Input: part model. Units: mm. Frame: model coordinates. A direction names the side the tool comes from. Round coordinates to 2 decimals unless told otherwise and drop trailing zeros. Loops run counter-clockwise (first coordinate to the right, second up) from the corner with the lowest first, then second, coordinate; pieces in that order, holes last.
1) Section A-A, the plane z = -59. Return loops of the section in (x, y), and give its area (3 significant figures).
2) Ray query, line 1 along Z through (x, y) = (-60.5, 0.5); line 2 along X through (y, z) = (-1, -37.5); line 3 along Z through (x, y) = (55.5, 4.75). Return the intervals inside material, ascending.
3) Section C-C, the plane y = -3.25. State how many separate pieces and enclosed holes the cut face has, and give its area (3 significant figures).
4) Draft query along Z for faces 1 (the face through (42, 4, -31)), 2 (the face through (-14, 5, -61)), 3 (the face through (-16, 6.25, -51)). Return one class per face: pulls with the +Z half, pulls with the -Z half, needs draft (parallel to the pull), parting line crosses it, or undercut.
5) First-contact query: pin 1 (4 mm diameter, centred on x = 57.5, y = 6.5, fed in from -Z); pin 2 (10 mm diameter, centred on x = -5.5, y = -2, fed in from +Z); pin 3 (2 mm diameter, centred on x = 34.5, z = -3, fed in from +Y). Flat tips, straight axial feed; report the tip coordinate or a pass-through.
6) Section D-D, the plane x = -1.5. Return loops of the section in (y, z).
7) Access query for faces 4 (the face through (-51.5, -1, 36)), 5 (the face through (48.95, 7, -30)), 6 (the face through (-11, 4, -66)). Directions: +Z, -Z, +X, -X, +Y, -Y. A direction counts if a zero-diameter tool reaches every point of the face in a straight line with its end or side. Return the directions, or none.
8) Section B-B, the plane x = 55.5. Return loops of the section in (y, z), and give its area (3 significant figures).
from build123d import *

# Parameters (mm, degrees)
SKETCH1_W           = 141
SKETCH1_H           = 82
BOSS_EXTRUDE1_DEPTH = 9
SKETCH3_R           = 2
CUT_EXTRUDE1_DEPTH  = 19
SKETCH4_W           = 8.7
SKETCH4_H           = 13.5
CUT_EXTRUDE2_DEPTH  = 10
SKETCH5_W           = 20
SKETCH5_H           = 5
CUT_EXTRUDE3_DEPTH  = 10
SKETCH6_W           = 3.23
SKETCH6_H           = 5.77
BOSS_EXTRUDE2_DEPTH = 3.3
SKETCH7_R           = 2.425
BOSS_EXTRUDE3_DEPTH = 20
LPATTERN1_COUNT     = 3
LPATTERN1_PITCH     = 31.7
SKETCH8_W           = 8.5
SKETCH8_H           = 5
SKETCH8_H_2         = 0.25
BOSS_EXTRUDE4_DEPTH = 30
SKETCH10_R          = 2.225
BOSS_EXTRUDE6_DEPTH = 5
LPATTERN2_COUNT     = 3
LPATTERN2_PITCH     = 31
SKETCH9_W           = 12
SKETCH9_H           = 5
SKETCH9_W_2         = 10
SKETCH9_W_3         = 5
SKETCH9_H_2         = 8
SKETCH9_H_3         = 18.5
SKETCH9_H_4         = 16.5
SKETCH9_W_4         = 8.75
SKETCH9_W_5         = 14
CUT_EXTRUDE4_DEPTH  = 5


with BuildPart() as part:
    # Sketch1 → Boss-Extrude1 (new body, symmetric)
    with BuildSketch(Plane(origin=(0, 0, 0), x_dir=(1, 0, 0), z_dir=(0, 1, 0))):
        Rectangle(SKETCH1_W, SKETCH1_H)
    extrude(amount=BOSS_EXTRUDE1_DEPTH, both=True)

    # Sketch3 → Cut-Extrude1 (cut, through all)
    with BuildSketch(Plane(origin=(0, 9, 0), x_dir=(1, 0, 0), z_dir=(0, 1, 0))):
        with Locations((-60.5, 37.5)):
            Circle(SKETCH3_R)
        with Locations((-1.5, 37.5)):
            Circle(SKETCH3_R)
        with Locations((55.5, 37.5)):
            Circle(SKETCH3_R)
    cut_extrude1 = extrude(amount=-CUT_EXTRUDE1_DEPTH, mode=Mode.SUBTRACT)

    # Mirror1: Cut-Extrude1 across plane
    add(cut_extrude1.mirror(Plane.XY), mode=Mode.SUBTRACT)

    # Sketch4 → Cut-Extrude2 (cut)
    with BuildSketch(Plane.XY.offset(41)):
        with Locations((-47.15, -0.75)):
            Rectangle(SKETCH4_W, SKETCH4_H)
        with Locations((-15.45, -0.75)):
            Rectangle(SKETCH4_W, SKETCH4_H)
        with Locations((16.25, -0.75)):
            Rectangle(SKETCH4_W, SKETCH4_H)
    extrude(amount=-CUT_EXTRUDE2_DEPTH, mode=Mode.SUBTRACT)

    # Sketch5 → Cut-Extrude3 (cut)
    with BuildSketch(Plane(origin=(0, 0, -41), x_dir=(-1, 0, 0), z_dir=(0, 0, -1))):
        with Locations((47, 3.5)):
            Rectangle(SKETCH5_W, SKETCH5_H)
        with Locations((16, 3.5)):
            Rectangle(SKETCH5_W, SKETCH5_H)
        with Locations((-15, 3.5)):
            Rectangle(SKETCH5_W, SKETCH5_H)
    extrude(amount=-CUT_EXTRUDE3_DEPTH, mode=Mode.SUBTRACT)

    # Sketch6 → Boss-Extrude2 (add)
    with BuildSketch(Plane(origin=(0, 9, 0), x_dir=(1, 0, 0), z_dir=(0, 1, 0))):
        with Locations((63.885, -23)):
            Rectangle(SKETCH6_W, SKETCH6_H)
        with BuildLine():
            Line((62.27, -20.115), (65.5, -20.115))
            ThreePointArc((65.5, -20.115), (63.885, -18.5), (62.27, -20.115))
        make_face()
        with BuildLine():
            ThreePointArc((65.5, -25.885), (63.885, -27.5), (62.27, -25.885))
            Line((62.27, -25.885), (65.5, -25.885))
        make_face()
    extrude(amount=BOSS_EXTRUDE2_DEPTH)

    # Sketch7 → Boss-Extrude3 (add)
    with BuildSketch(Plane.XY.offset(31)):
        with Locations((-47.15, 1.75)):
            Circle(SKETCH7_R)
        with Locations((-47.15, -3.25)):
            Circle(SKETCH7_R)
    boss_extrude3 = extrude(amount=BOSS_EXTRUDE3_DEPTH)

    # LPattern1: Boss-Extrude3 ×3
    with Locations(*[(i * LPATTERN1_PITCH, 0, 0) for i in range(1, LPATTERN1_COUNT)]):
        add(boss_extrude3)

    # Sketch8 → Boss-Extrude4 (add)
    with BuildSketch(Plane(origin=(0, 0, -31), x_dir=(-1, 0, 0), z_dir=(0, 0, -1))):
        with Locations((47, 3.5)):
            Rectangle(SKETCH8_W, SKETCH8_H)
        with BuildLine():
            Line((51.25, 6), (51.25, 1))
            Line((51.25, 1), (52.395643924, 1))
            ThreePointArc((52.395643924, 1), (54, 3.5), (52.395643924, 6))
            Line((52.395643924, 6), (51.25, 6))
        make_face()
        with BuildLine():
            Line((41.604356076, 1), (42.75, 1))
            Line((42.75, 1), (42.75, 6))
            Line((42.75, 6), (41.604356076, 6))
            ThreePointArc((41.604356076, 6), (40, 3.5), (41.604356076, 1))
        make_face()
        with Locations((47, 6.125)):
            Rectangle(SKETCH8_W, SKETCH8_H_2)
        with BuildLine():
            Line((51.25, 6.25), (51.25, 6))
            Line((51.25, 6), (52.395643924, 6))
            ThreePointArc((52.395643924, 6), (51.83630197, 6.186773158), (51.25, 6.25))
        make_face()
        with BuildLine():
            Line((41.604356076, 6), (42.75, 6))
            Line((42.75, 6), (42.75, 6.25))
            ThreePointArc((42.75, 6.25), (42.16369803, 6.186773158), (41.604356076, 6))
        make_face()
        with BuildLine():
            ThreePointArc((41.604356076, 1), (42.16369803, 0.813226842), (42.75, 0.75))
            Line((42.75, 0.75), (42.75, 1))
            Line((42.75, 1), (41.604356076, 1))
        make_face()
        with Locations((47, 0.875)):
            Rectangle(SKETCH8_W, SKETCH8_H_2)
        with BuildLine():
            Line((51.25, 1), (51.25, 0.75))
            ThreePointArc((51.25, 0.75), (51.83630197, 0.813226842), (52.395643924, 1))
            Line((52.395643924, 1), (51.25, 1))
        make_face()
    boss_extrude4 = extrude(amount=BOSS_EXTRUDE4_DEPTH)

    # Sketch10 → Boss-Extrude6 (add)
    with BuildSketch(Plane(origin=(0, 0, -61), x_dir=(-1, 0, 0), z_dir=(0, 0, -1))):
        with Locations((51.5, 3.5)):
            Circle(SKETCH10_R)
        with Locations((47, 3.5)):
            Circle(SKETCH10_R)
        with Locations((42.5, 3.5)):
            Circle(SKETCH10_R)
    boss_extrude6 = extrude(amount=BOSS_EXTRUDE6_DEPTH)

    # LPattern2: Boss-Extrude4, Boss-Extrude6 ×3
    with Locations(*[(i * LPATTERN2_PITCH, 0, 0) for i in range(1, LPATTERN2_COUNT)]):
        add(boss_extrude4)
        add(boss_extrude6)

    # Sketch9 → Cut-Extrude4 (cut)
    with BuildSketch(Plane(origin=(0, 9, 0), x_dir=(1, 0, 0), z_dir=(0, 1, 0))):
        with Locations((44.2, -30)):
            Rectangle(SKETCH9_W, SKETCH9_H)
        with Locations((55.5, -30)):
            Rectangle(SKETCH9_W_2, SKETCH9_H)
        with Locations((64, -10.8)):
            Rectangle(SKETCH9_W_3, SKETCH9_H_2)
        with Locations((64, 2.75)):
            Rectangle(SKETCH9_W_3, SKETCH9_H_3)
        with Locations((64, 22.75)):
            Rectangle(SKETCH9_W_3, SKETCH9_H_4)
        with Locations((53.625, 30.5)):
            Rectangle(SKETCH9_W_4, SKETCH9_H)
        with Locations((41.95, 30.5)):
            Rectangle(SKETCH9_W_5, SKETCH9_H)
    extrude(amount=-CUT_EXTRUDE4_DEPTH, mode=Mode.SUBTRACT)


solid = part.part
Final values:
1. outline: (-51.25, 0.75) - (-42.75, 0.75) arc R2.75 ccw to (-42.75, 6.25) - (-51.25, 6.25) arc R2.75 ccw to start; (-20.25, 0.75) - (-11.75, 0.75) arc R2.75 ccw to (-11.75, 6.25) - (-20.25, 6.25) arc R2.75 ccw to start; (10.75, 0.75) - (19.25, 0.75) arc R2.75 ccw to (19.25, 6.25) - (10.75, 6.25) arc R2.75 ccw to start
1. area: 212 mm2
2. line 1: z = -41 to -39.5, -35.5 to 35.5, 39.5 to 41
2. line 2: x = -70.5 to -62.5, -58.5 to -3.5, 0.5 to 53.5, 57.5 to 70.5
2. line 3: z = -41 to -39.5, -35.5 to -33, -28 to 27.5, 32.5 to 35.5, 39.5 to 41
3. separate pieces: 1
3. enclosed holes: 6
3. area: 11,500 mm2
4. face 1: undercut
4. face 2: pulls with the -Z half
4. face 3: needs draft
5. pin 1: stops at z = -41
5. pin 2: stops at z = 41
5. pin 3: stops at y = 9
6. outline: (-9, -41) - (9, -41) - (9, -39.5) - (-9, -39.5) - close; (-9, -35.5) - (9, -35.5) - (9, 35.5) - (-9, 35.5) - close; (-9, 39.5) - (9, 39.5) - (9, 41) - (-9, 41) - close
7. face 4: +Z
7. face 5: +Y
7. face 6: -Z, +X, -X, +Y, -Y
8. outline: (-9, -41) - (9, -41) - (9, -39.5) - (-9, -39.5) - close; (-9, -35.5) - (9, -35.5) - (9, -33) - (4, -33) - (4, -28) - (9, -28) - (9, 27.5) - (4, 27.5) - (4, 32.5) - (9, 32.5) - (9, 35.5) - (-9, 35.5) - close; (-9, 39.5) - (9, 39.5) - (9, 41) - (-9, 41) - close
8. area: 1,280 mm2
